from build123d import *

# Parameters (mm, degrees)
SKETCH_1_W          = 60
SKETCH_1_H          = 50
EXTRUDE_1_DEPTH     = 5
HOLE_WIZARD_1_D     = 9.5
HOLE_WIZARD_1_DEPTH = 20
CHAMFER_1_SIZE      = 4
SKETCH_15_R         = 1.6
CUT_EXTRUDE_1_DEPTH = 40.37003937
HOLE_WIZARD_2_D     = 8.2
SKETCH_19_W         = 2.7
SKETCH_19_H         = 6
CUT_EXTRUDE_2_DEPTH = 10
HOLE_WIZARD_3_D     = 3.2
HOLE_WIZARD_3_DEPTH = 10


with BuildPart() as part:
    # 草图1 → 凸台-拉伸1 (new body)
    with BuildSketch(Plane.XY):
        Rectangle(SKETCH_1_W, SKETCH_1_H)
    extrude(amount=EXTRUDE_1_DEPTH)

    # 孔1
    with Locations(Plane.XY.offset(5)):
        with Locations((0, 0)):
            Hole(HOLE_WIZARD_1_D / 2, depth=HOLE_WIZARD_1_DEPTH)

    # 倒角1
    chamfer_1_edges = [part.edges().sort_by_distance(p)[0] for p in [
        (30, -25, 2.5),
        (-30, -25, 2.5),
        (-30, 25, 2.5),
        (30, 25, 2.5),
    ]]
    chamfer(chamfer_1_edges, length=CHAMFER_1_SIZE)

    # 草图15 → 切除-拉伸1 (cut, through all)
    with BuildSketch(Plane.XY.offset(5)):
        with BuildLine():
            ThreePointArc((-21.13137085, 21.13137085), (-21.13137085, 18.86862915), (-18.86862915, 18.86862915))
            Line((-18.86862915, 18.86862915), (-21.13137085, 21.13137085))
        make_face()
        with BuildLine():
            Line((-21.13137085, 21.13137085), (-18.86862915, 18.86862915))
            ThreePointArc((-18.86862915, 18.86862915), (-18.521792748, 19.387706508), (-18.4, 20))
            ThreePointArc((-18.4, 20), (-19.387706508, 21.478207252), (-21.13137085, 21.13137085))
        make_face()
        with Locations((20, 20)):
            Circle(SKETCH_15_R)
        with Locations((20, -20)):
            Circle(SKETCH_15_R)
        with Locations(Location((-20, -20, 0), (0, 0, 180))):
            Circle(SKETCH_15_R)
    extrude(amount=-CUT_EXTRUDE_1_DEPTH, mode=Mode.SUBTRACT)

    # 孔2 (through all)
    with Locations(Plane.XY.offset(5)):
        with Locations((-20, 0), (20, 0)):
            Hole(HOLE_WIZARD_2_D / 2)

    # 草图19 → 切除-拉伸2 (cut)
    with BuildSketch(Plane.XY.offset(5)):
        with Locations((27.05, 0)):
            Rectangle(SKETCH_19_W, SKETCH_19_H)
    cut_extrude_2 = extrude(amount=-CUT_EXTRUDE_2_DEPTH, mode=Mode.SUBTRACT)

    # 孔3
    with Locations(Plane(origin=(30, 0, 0), x_dir=(0, 0, -1), z_dir=(1, 0, 0))):
        with Locations((-2.5, 0)):
            hole_wizard_3 = Hole(HOLE_WIZARD_3_D / 2, depth=HOLE_WIZARD_3_DEPTH)

    # 镜向1: 切除-拉伸2, 孔3 across plane
    add(cut_extrude_2.mirror(Plane(origin=(0, 0, 0), x_dir=(0, 0, 1), z_dir=(1, 0, 0))), mode=Mode.SUBTRACT)
    add(hole_wizard_3.mirror(Plane(origin=(0, 0, 0), x_dir=(0, 0, 1), z_dir=(1, 0, 0))), mode=Mode.SUBTRACT)


solid = part.part
Geometry check sheet. Reference: the model listing, model coordinates, mm. A direction names the side the tool comes from. Give positions to 0.01 mm unless a question says otherwise; leave off trailing zeros. Write each loop counter-clockwise with the first axis right and the second up, starting at its lowest first coordinate (ties: lowest second). Pieces come first, ordered by that corner, then holes.
1) Set-up check for faces 1 (the face through (-27, 3, 3)), 2 (the face through (-28, -23, 2)), 3 (the face through (29.19, 0.07, 0.9)), 4 (the face through (0, 6, 5)), 5 (the face through (-24.72, -0.61, 3.98)): record each of +Z, -Z, +X, -X, +Y, -Y from which the full face is reachable in a straight line by a thin tool's end or side.
Values follow:
face 1: +Z, -Z
face 2: +Z, -Z, -X, -Y
face 3: +X
face 4: +Z, +X, -X, +Y, -Y
face 5: -X
2) Cross-section at C-C (x = 0). Record the boundary of the cut face in (y, z).
Values follow:
outline: (-25, 0) - (-4.75, 0) - (-4.75, 5) - (-25, 5) - close; (4.75, 0) - (25, 0) - (25, 5) - (4.75, 5) - close
3) Cross-section at D-D (z = 2.5). Count the separate pieces of the cut face and the enclosed holes in it, plus the area to 3 significant figures.
Values follow:
separate pieces: 1
enclosed holes: 5
area: 2,710 mm2
4) Cross-section at B-B (y = -20). Record the boundary of the cut face in (x, z).
Values follow:
outline: (-30, 0) - (-21.6, 0) - (-21.6, 5) - (-30, 5) - close; (-18.4, 0) - (18.4, 0) - (18.4, 5) - (-18.4, 5) - close; (21.6, 0) - (30, 0) - (30, 5) - (21.6, 5) - close
5) Thickness scan on line 1 (Y direction, x = 20, z = 3.55); line 2 (Y direction, x = -20.5, z = 3.25); line 3 (Y direction, x = 2, z = 0.25). Record the ranges inside material, lowest first.
Values follow:
line 1: y = -25 to -21.6, -18.4 to -4.1, 4.1 to 18.4, 21.6 to 25
line 2: y = -25 to -21.52, -18.48 to -4.07, 4.07 to 18.48, 21.52 to 25
line 3: y = -25 to -4.31, 4.31 to 25
6) Go/stop test with flat-tipped pins: pin 1 Ø0.8 at (x, z) = (-27, 2.5) entering from -Y; pin 2 Ø3 at (y, z) = (0, 2.5) entering from -X. Record where each tip stops, or that it passes through.
Values follow:
pin 1: stops at y = -24.4
pin 2: stops at x = -16.18
7) Cross-section at A-A (x = -20). Record the boundary of the cut face in (y, z).
Values follow:
outline: (-25, 0) - (-21.6, 0) - (-21.6, 5) - (-25, 5) - close; (-18.4, 0) - (-4.1, 0) - (-4.1, 5) - (-18.4, 5) - close; (4.1, 0) - (18.4, 0) - (18.4, 5) - (4.1, 5) - close; (21.6, 0) - (25, 0) - (25, 5) - (21.6, 5) - close
8) Release check for a two-part mould opening along X. For faces 6 (the face through (-30, -0.3, 4.7)), 7 (the face through (25.7, 1, 4)), 8 (the face through (16.213, -1.57, 2.465)), 9 (the face through (0, -25, 2)) record: released by +X, released by -X, zero draft, split by the parting line, or undercut.
Values follow:
face 6: released by -X
face 7: undercut
face 8: undercut
face 9: zero draft
